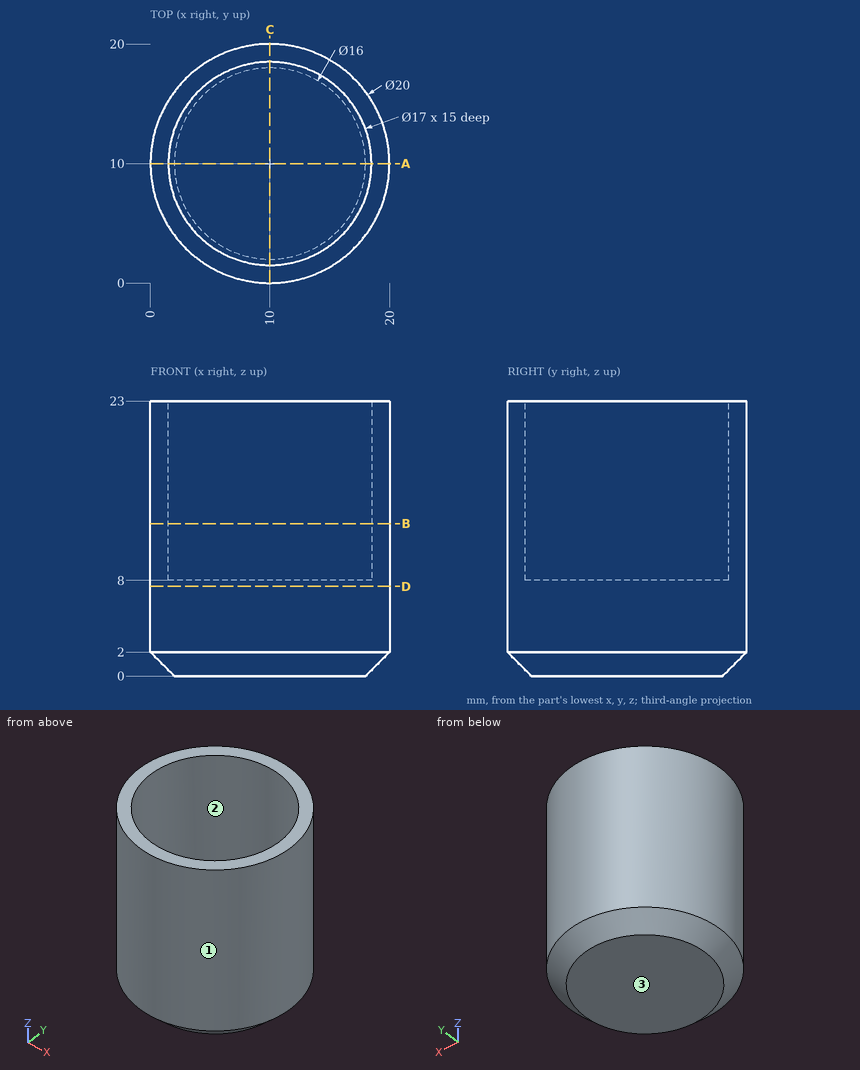
For this review, use the dimensioned drawing (mm, ordinates from the lowest corner) and the shaded views. Give positions to 0.01 mm unless a question says otherwise; leave off trailing zeros. Order: outer loops, then holes, each group sorted by start corner. A loop starts at its lowest first (then second) coordinate and runs counter-clockwise, first axis right, second up. Notation, with made-up numbers: M 74.25,-39 L 97.25,-39 A20 ccw 97.25,-14 Z; hole C -33.5,42.25 d9. An arc over 180 degrees is marked long. Use one line per item in the form item = value. Start each with the question number.
Item 1: We need section A-A on y = 10. Give the boundary of the cut face in (x, z).
Item 2: The part is to be moulded in two halves that separate along Y. For the marked faces 1, 2 and 3, say which applies: pulls with the +Y half, pulls with the -Y half, needs draft (parallel to the pull), parting line crosses it, or undercut.
Item 3: We need section B-B on z = 12.75. Give the boundary of the cut face in (x, y).
Item 4: To check wall thickness, follow line 1 along Y through (x, z) = (10, 13.25); line 2 along X through (y, z) = (4.25, 20.5); line 3 along Y through (x, z) = (11, 13). State the ranges of each line that lie inside material, in increasing order. Write a range as from..to.
Item 5: Insertion check: pin 1 Ø10 at (x, y) = (10, 10) entering from +Z; pin 2 Ø10 at (y, z) = (3.5, 13.5) entering from +X; pin 3 Ø6 at (x, z) = (16.5, 17) entering from -Y. Each pin has a flat end and moves straight along its axis. Give the tip position at first contact, or say it passes through.
Item 6: We need section D-D on z = 7.5. Give the boundary of the cut face in (x, y), plus the area to 3 significant figures.
Completed:
q1.outline = M 0,2 L 2,0 L 18,0 L 20,2 L 20,23 L 18.5,23 L 18.5,8 L 1.5,8 L 1.5,23 L 0,23 Z
q2.face_1 = parting line crosses it
q2.face_2 = undercut
q2.face_3 = needs draft
q3.outline = C 10,10 d20; hole C 10,10 d17
q4.line_1 = 0..1.5, 18.5..20
q4.line_2 = 1.82..3.74, 16.26..18.18
q4.line_3 = 0.05..1.56, 18.44..19.95
q5.pin_1 = 8
q5.pin_2 = 19.89
q5.pin_3 = 0.63
q6.outline = C 10,10 d20
q6.area = 314 mm²
